Can you work these out from the model? Positions are in its coordinate system, mm. Coordinates: 2 decimals unless noted, no trailing zeros. Order: outer loops, then holes, each group sorted by start corner. A loop starts at its lowest first (then second) coordinate and runs counter-clockwise, first axis right, second up. Notation, with made-up numbers: (18, -25.75) -> (69, -25.75) arc R13 ccw to (69, -10.75) -> close; hole circle Ø6 at (8.5, 55.5). An arc over 180 degrees is marked (long way). Write item = value, one per line. Start each with the question number.
Autodesk Inventor part; units mm, degrees
ref_plane "YZ Plane" through (0, 0, 0) normal (1, 0, 0) x (0, 1, 0)
ref_plane "XZ Plane" through (0, 0, 0) normal (0, 1, 0) x (-1, 0, 0)
ref_plane "XY Plane" through (0, 0, 0) normal (0, 0, 1) x (1, 0, 0)
sketch "Sketch1" plane through (0, 0, 0) normal (0, 0, 1) x (1, 0, 0)
  line L0 (0, 0) -> (213.35, 0)
  line L1 (213.35, 0) -> (213.35, 266.7)
  line L2 (213.35, 266.7) -> (0, 266.7)
  line L3 (0, 266.7) -> (0, 0)
  line L4 (0, 0) -> (41.275, 0)
  line L5 (0, 41.275) -> (0, 0)
  line L6 (0, 266.7) -> (40, 266.7)
  line L7 (40, 266.7) -> (40, 226.7)
  line L8 (40, 226.7) -> (0, 226.7)
  line L9 (0, 226.7) -> (0, 266.7)
  dimension "d0" = 266.7
  dimension "d1" = 213.35
  dimension "d4" = 40
extrude "Extrusion1" add sketch "Sketch1" along normal blind 1.5875 contours L3 L8 L7 L2 L1 L0
sketch "Sketch2" plane through (0, 0, 1.5875) normal (0, 0, 1) x (1, 0, 0)
  line L0 (213.35, 0) -> (0, 0)
  line L1 (213.35, 266.7) -> (213.35, 0)
  line L2 (40, 266.7) -> (213.35, 266.7)
  line L3 (20, 189.55) -> (20, 37.15)
  line L4 (40, 266.7) -> (40, 226.7)
  line L5 (40, 266.7) -> (213.35, 266.7)
  line L6 (0, 0) -> (0, 226.7)
  line L7 (0, 226.7) -> (40, 226.7)
  line L8 (213.35, 266.7) -> (213.35, 0)
  line L9 (193.35, 215.9) -> (193.35, 63.5)
  point P0 (41.275, 0)
  point P1 (126.675, 266.7)
  point P2 (20, 113.35)
  point P3 (0, 113.35)
  dimension "d9" = 152.4
  dimension "d19" = 20
  dimension "d20" = 20
  dimension "d21" = 152.4
  dimension "d22" = 50.8
hole "Mounting Holes" at (20, 189.55, 1.5875) at (20, 37.15, 1.5875) at (193.35, 215.9, 1.5875) at (193.35, 63.5, 1.5875) direction (0, 0, -1) diameter 8.9916 end through all
sketch "Sketch3" plane through (0, 0, 0) normal (0, 0, -1) x (-1, 0, 0)
  line L0 (-213.35, 0) -> (-213.35, 266.7)
  line L1 (0, 0) -> (-213.35, 0)
  line L2 (0, 226.7) -> (-40, 226.7)
  line L3 (-108.575, 196.85) -> (-108.575, 38.1)
  dimension "d23" = 104.775
  dimension "d24" = 158.75
  dimension "d25" = 38.1
hole "DIN Rail Holes" at (108.575, 196.85, 0) at (108.575, 38.1, 0) direction (0, 0, 1) diameter 4.4958 end through all
properties part number "front left plate" material "Aluminum-6061"
(1) Imagine slicing it at B-B (x = 20). Write out the boundary of the cut face in (y, z), plus the area to 3 significant figures.
(2) Imagine slicing it at A-A (y = 189.55). Write out the boundary of the cut face in (x, z), plus the area to 3 significant figures.
(3) Thinking about a two-plate mould opening in Y: for faces 1 (the face through (197.74, 64.47, 0.78)), 2 (the face through (105, 135, 0)), which applies, +Y half, -Y half, draft (parallel to the pull), parting line (faces both ways), or undercut?
(4) For P1, Ø0.8, axis at y = 251.5, z = 1, coming from the -X side; P2, Ø7, axis at x = 20, y = 37.15, coming from the +Z side, each with a flat end and sliding along its axis, tell me the tip position at first contact or that it passes through.
(5) Imagine slicing it at D-D (z = 0.95). Write out the boundary of the cut face in (x, y) (3 decimals), plus the area to 3 significant figures.
(6) Imagine slicing it at C-C (x = 193.35). Write out the boundary of the cut face in (y, z), plus the area to 3 significant figures.
(7) If I drill on L1, parallel to Y at x = 20, z = 0.75; L2, parallel to X at y = 63.5, z = 0.8; L3, parallel to X at y = 196.85, z = 0.5, over which ranges is the centre line in solid material (lowest first)? Write a range as from..to.
Result set:
q1.outline = (0, 0) -> (32.65, 0) -> (32.65, 1.59) -> (0, 1.59) -> close; (41.65, 0) -> (185.05, 0) -> (185.05, 1.59) -> (41.65, 1.59) -> close; (194.05, 0) -> (226.7, 0) -> (226.7, 1.59) -> (194.05, 1.59) -> close
q1.area = 331 mm2
q2.outline = (0, 0) -> (15.5, 0) -> (15.5, 1.59) -> (0, 1.59) -> close; (24.5, 0) -> (213.35, 0) -> (213.35, 1.59) -> (24.5, 1.59) -> close
q2.area = 324 mm2
q3.face_1 = undercut
q3.face_2 = draft
q4.P1 = 40
q4.P2 = through
q5.outline = (0, 0) -> (213.35, 0) -> (213.35, 266.7) -> (40, 266.7) -> (40, 226.7) -> (0, 226.7) -> close; hole circle Ø8.992 at (20, 37.15); hole circle Ø8.992 at (20, 189.55); hole circle Ø4.496 at (108.575, 38.1); hole circle Ø4.496 at (108.575, 196.85); hole circle Ø8.992 at (193.35, 63.5); hole circle Ø8.992 at (193.35, 215.9)
q5.area = 55,000 mm2
q6.outline = (0, 0) -> (59, 0) -> (59, 1.59) -> (0, 1.59) -> close; (68, 0) -> (211.4, 0) -> (211.4, 1.59) -> (68, 1.59) -> close; (220.4, 0) -> (266.7, 0) -> (266.7, 1.59) -> (220.4, 1.59) -> close
q6.area = 395 mm2
q7.L1 = 0..32.65, 41.65..185.05, 194.05..226.7
q7.L2 = 0..188.85, 197.85..213.35
q7.L3 = 0..106.33, 110.82..213.35
